Input: part model. Units: mm. Frame: model coordinates. A direction names the side the tool comes from. Give positions to 0.01 mm unless a question says otherwise; leave off trailing zeros. Order: outer loops, then holes, each group sorted by start corner. A loop starts at its lowest first (then second) coordinate and runs counter-clockwise, first axis right, second up.
```python
from build123d import *

# Parameters (mm, degrees)
F0_W      = 1348.74
F0_H      = 685.8
F1_DEPTH  = 25.4
F4_W      = 50.8
F4_H      = 317.5
F5_DEPTH  = 9.525
F7_W      = 50.8
F7_H      = 76.2
F8_DEPTH  = 688.34
F10_DEPTH = 25.4
F12_DEPTH = 25.4
F13_W     = 1183.64
F13_H     = 8.255
F14_DEPTH = 307.975


with BuildPart() as f1:
    # F0 (on Top) → F1 (new body)
    with BuildSketch(Plane.XY):
        with Locations((15.8387869596, 66.6778717405)):
            Rectangle(F0_W, F0_H)
    extrude(amount=-F1_DEPTH)

    # F4 (on face) → F5 (join)
    with BuildSketch(Plane.XY):
        with Locations((-601.3812130404, 120.6528717405)):
            Rectangle(F4_W, F4_H)
        with Locations((633.0587869596, 120.6528717405)):
            Rectangle(F4_W, F4_H)
    extrude(amount=F5_DEPTH)

    # F7 (on face) → F8 (join)
    with BuildSketch(Plane.XY):
        with Locations((-601.7126866341, -76.1971282595)):
            Rectangle(F7_W, F7_H)
        with Locations((633.0587869596, -76.1971282595)):
            Rectangle(F7_W, F7_H)
    extrude(amount=F8_DEPTH)

    # F9 (on face) → F10 (join)
    with BuildSketch(Plane.XY.offset(688.34)):
        with BuildLine():
            ThreePointArc((-601.7126866341, -212.7221282595), (-583.7521743919, -205.2826405017), (-576.3126866341, -187.3221282595))
            Line((-576.3126866341, -187.3221282595), (-576.3126866341, 320.6778717405))
            ThreePointArc((-576.3126866341, 320.6778717405), (-583.7521743919, 338.6383839826), (-601.7126866341, 346.0778717405))
            ThreePointArc((-601.7126866341, 346.0778717405), (-619.6731988762, 338.6383839826), (-627.1126866341, 320.6778717405))
            Line((-627.1126866341, 320.6778717405), (-627.1126866341, -187.3221282595))
            ThreePointArc((-627.1126866341, -187.3221282595), (-619.6731988762, -205.2826405017), (-601.7126866341, -212.7221282595))
        make_face()
    extrude(amount=F10_DEPTH)

    # F11 (on face) → F12 (join)
    with BuildSketch(Plane.XY.offset(688.34)):
        with BuildLine():
            ThreePointArc((607.6587869596, -212.7221282595), (633.0587869596, -238.1221282595), (658.4587869596, -212.7221282595))
            Line((658.4587869596, -212.7221282595), (658.4587869596, 295.2778717405))
            ThreePointArc((658.4587869596, 295.2778717405), (651.0192992018, 313.2383839826), (633.0587869596, 320.6778717405))
            ThreePointArc((633.0587869596, 320.6778717405), (615.0982747175, 313.2383839826), (607.6587869596, 295.2778717405))
            Line((607.6587869596, 295.2778717405), (607.6587869596, -212.7221282595))
        make_face()
    extrude(amount=F12_DEPTH)

    # F13 (on face) → F14 (join)
    with BuildSketch(Plane.XY):
        with Locations((15.8387869596, -110.1696282595)):
            Rectangle(F13_W, F13_H)
    extrude(amount=F14_DEPTH)


solid = f1.part
```
1) Cut plane D-D (x = -50.5). Return the cut outline in (y, z) (3 decimals), then the cut area to 3 significant figures.
2) First-contact query: P1, Ø6.5, axis at x = -58, y = -109.5, coming from the +Z side (3 decimals); P2, Ø3, axis at x = -612, z = 6.5, coming from the +Y side; P3, Ø2, axis at x = 29.5, y = 166, coming from the +Z side. Flat tips, straight axial feed; report the tip coordinate or a pass-through.
3) Cut plane B-B (y = 162). Return the cut outline in (x, z) (3 decimals).
4) Cut plane A-A (z = 471.5). Return the cut outline in (x, y).
5) Line query: probe 1 along Z at (x, y) = (24, 43.5); probe 2 along Y at (x, z) = (-326, 183). Output: solid intervals per line, ascending.
6) Reachability of faces 1 (the face through (633, 144, 688.34)), 2 (the face through (607.659, -52, 461)), 3 (the face through (-602, -163, 688.34)) from +Z, -Z, +X, -X, +Y, -Y: full face, straight path, thin tool, end or side. Return the list, or none.
7) Pull-direction query (X, two-part tool) for faces 4 (the face through (6, 71, 0)), 5 (the face through (-602, 157, 688.34)), 6 (the face through (690.209, 62, -13)); classes: pulls with the +X half, pulls with the -X half, needs draft (parallel to the pull), parting line crosses it, or undercut.
8) Cut plane C-C (z = 147). Return the cut outline in (x, y).
Geometry says:
1. outline: (-276.222, -25.4) - (409.578, -25.4) - (409.578, 0) - (-106.042, 0) - (-106.042, 307.975) - (-114.297, 307.975) - (-114.297, 0) - (-276.222, 0) - close
1. area: 20,000 mm2
2. P1: stops at z = 307.975
2. P2: stops at y = 279.4
2. P3: stops at z = 0
3. outline: (-658.531, -25.4) - (690.209, -25.4) - (690.209, 0) - (658.459, 0) - (658.459, 9.525) - (607.659, 9.525) - (607.659, 0) - (-575.981, 0) - (-575.981, 9.525) - (-626.781, 9.525) - (-626.781, 0) - (-658.531, 0) - close; (-627.113, 688.34) - (-576.313, 688.34) - (-576.313, 713.74) - (-627.113, 713.74) - close; (607.659, 688.34) - (658.459, 688.34) - (658.459, 713.74) - (607.659, 713.74) - close
4. outline: (-627.11, -114.3) - (-576.31, -114.3) - (-576.31, -38.1) - (-627.11, -38.1) - close; (607.66, -114.3) - (658.46, -114.3) - (658.46, -38.1) - (607.66, -38.1) - close
5. probe 1: z = -25.4 to 0
5. probe 2: y = -114.3 to -106.04
6. face 1: +X, -X, +Y
6. face 2: +Z, +Y
6. face 3: +X, -X, -Y
7. face 4: undercut
7. face 5: needs draft
7. face 6: pulls with the +X half
8. outline: (-627.11, -114.3) - (-576.31, -114.3) - (-576.31, -38.1) - (-627.11, -38.1) - close; (-575.98, -114.3) - (658.46, -114.3) - (658.46, -38.1) - (607.66, -38.1) - (607.66, -106.04) - (-575.98, -106.04) - close
